from build123d import *

# Parameters (mm, degrees)
EXTRUDE_1_DEPTH = 10
SKETCH_5_R      = 6
EXTRUDE_2_DEPTH = 10


with BuildPart() as part:
    # 草图1 → 凸台-拉伸1 (new body)
    with BuildSketch(Plane(origin=(0, 0, 0), x_dir=(1, 0, 0), z_dir=(0, 1, 0))):
        with BuildLine():
            Line((-30, 30), (30, 30))
            ThreePointArc((30, 30), (37.071067812, 27.071067812), (40, 20))
            Line((40, 20), (40, -20))
            ThreePointArc((40, -20), (37.071067812, -27.071067812), (30, -30))
            Line((30, -30), (-30, -30))
            ThreePointArc((-30, -30), (-37.071067812, -27.071067812), (-40, -20))
            Line((-40, -20), (-40, 20))
            ThreePointArc((-40, 20), (-37.071067812, 27.071067812), (-30, 30))
        make_face()
    extrude(amount=EXTRUDE_1_DEPTH)

    # 草图5 → 凸台-拉伸2 (add)
    with BuildSketch(Plane(origin=(4.105168422, 1.435917424, 3.444645309), x_dir=(0.6427876096865377, 0, -0.7660444431189795), z_dir=(0.73994211169385, 0.2588190451025179, 0.6208851530148445))):
        with BuildLine():
            Line((-19.928849561, 8.866190698), (25.071150439, 8.866190698))
            Line((25.071150439, 8.866190698), (18.334609469, 47.607241481))
            ThreePointArc((18.334609469, 47.607241481), (2.571150439, 60.866190698), (-13.192308592, 47.607241481))
            Line((-13.192308592, 47.607241481), (-19.928849561, 8.866190698))
        make_face()
        with Locations((2.571150439, 44.866190698)):
            Circle(SKETCH_5_R, mode=Mode.SUBTRACT)
    extrude(amount=-EXTRUDE_2_DEPTH)


solid = part.part
CAD build for the part. Positions are in the model's coordinates, mm. Give positions to 0.01 mm unless a question says otherwise; leave off trailing zeros. Write each loop counter-clockwise with the first axis right and the second up, starting at its lowest first coordinate (ties: lowest second). Pieces come first, ordered by that corner, then holes. Notation, with made-up numbers: M -38,52.25 L -7,52.25 A19 cw -7,77.25 Z; hole C 23,22 d11. An arc over 180 degrees is marked long. Put each result on its own line as item: value. Start each with the question number.
(1) Band-saw the part on C-C, the plane z = 14.5. Write the cut outline in (x, y), and give its area (3 significant figures).
(2) Band-saw the part on D-D, the plane x = 13. Write the cut outline in (y, z), and give its area (3 significant figures).
(3) Band-saw the part on B-B, the plane x = 24.5. Write the cut outline in (y, z).
(4) Probe L1, parallel to Y at x = 23, z = 25; L2, parallel to X at y = 12.5, z = -20.5; L3, parallel to X at y = 52, z = -22.5. List the from-to ranges inside material, lowest first.
(5) Band-saw the part on A-A, the plane y = 5.5. Write the cut outline in (x, z).
(6) Flat gauge pins, fed straight in: pin 1 Ø3 at (x, z) = (24.5, -6.5) entering from +Y; pin 2 Ø3 at (x, z) = (-21.5, -9.5) entering from -Y; pin 3 Ø6 at (y, z) = (36.5, -21) entering from -X; pin 4 Ø8 at (x, y) = (2, 25.5) entering from +Z. Where does each tip first touch, or does it go through?
(7) Mould opens along Z. For faces 1 (the face through (-8, 28.86, -9.67)), 2 (the face through (-36.99, 4.93, 27.15)), 3 (the face through (-8.467, 49.244, -9.441)) say: +Z half, -Z half, draft (parallel to the pull), parting line (faces both ways), or undercut.
Response values:
1. outline: M -40,0 L 40,0 L 40,10 L -8.17,10 L -11.25,18.82 L -13.44,10 L -40,10 Z
1. area: 823 mm2
2. outline: M 0,-30 L 10,-30 L 10,-21.42 L 27.02,-17.82 L 10,-10.73 L 10,30 L 0,30 Z
2. area: 691 mm2
3. outline: M 0,-30 L 10,-30 L 10,30 L 0,30 Z
4. L1: y = 0 to 10
4. L2: x = 6.81 to 13.51
4. L3: x = -5.33 to -3.02
5. outline: M -40,-20 A10 ccw -30,-30 L 30,-30 A10 ccw 40,-20 L 40,20 A10 ccw 30,30 L -30,30 A10 ccw -40,20 Z
6. pin 1: stops at y = 10
6. pin 2: stops at y = 0
6. pin 3: stops at x = -3.89
6. pin 4: stops at z = 0.97
7. face 1: -Z half
7. face 2: +Z half
7. face 3: undercut
